Part model, mm, in its own coordinate system. A direction names the side the tool comes from. Round coordinates to 2 decimals unless told otherwise and drop trailing zeros. Loops run counter-clockwise (first coordinate to the right, second up) from the corner with the lowest first, then second, coordinate; pieces in that order, holes last. Notation, with made-up numbers: M -22.75,-1.75 L 9.25,-1.75 A18 cw 9.25,13.25 Z; hole C -14.5,68.25 d3. An arc over 180 degrees is marked long. Write each question's results on one line, items separated by ' | '.
from build123d import *

# Parameters (mm, degrees)
PROFILEBOSS_EXTRUDE1_DEPTH           = 270
SKETCH2_R                            = 2.3
LEDSTRIPMOUNTHOLESCUT_EXTRUDE1_DEPTH = 4.5
SKETCH3_R                            = 2.3
MOUNTINGHOLESCUT_EXTRUDE3_DEPTH      = 4.5
SKETCH4_W                            = 28
SKETCH4_H                            = 11.5
POWERCONNECTORCUT_EXTRUDE4_DEPTH     = 6.5


with BuildPart() as part:
    # Sketch1 → ProfileBoss-Extrude1 (new body)
    with BuildSketch(Plane(origin=(0, 0, 0), x_dir=(0, 0, -1), z_dir=(1, 0, 0))):
        with BuildLine():
            Line((0, 0), (2.499461553, 0))
            ThreePointArc((2.499461553, 0), (3.914055855, 0.585944145), (4.5, 2.000538447))
            Line((4.5, 2.000538447), (4.5, 3.5))
            Line((4.5, 3.5), (14.922539551, 8.36011001))
            Line((14.922539551, 8.36011001), (16.190394336, 5.641186649))
            ThreePointArc((16.190394336, 5.641186649), (17.700753359, 6.16912635), (18.340729536, 7.635528477))
            Line((18.340729536, 7.635528477), (18.340729536, 13.36011001))
            ThreePointArc((18.340729536, 13.36011001), (17.754943098, 14.774323572), (16.340729536, 15.36011001))
            Line((16.340729536, 15.36011001), (0, 15.36011001))
            Line((0, 15.36011001), (0, 0))
        make_face()
    extrude(amount=PROFILEBOSS_EXTRUDE1_DEPTH)

    # Sketch2 → LedStripMountHolesCut-Extrude1 (cut)
    with BuildSketch(Plane(origin=(0, 1.15127832, 0.536849897), x_dir=(1, 0, 0), z_dir=(0, -0.906307787036651, -0.4226182617406973))):
        with Locations(Location((36.15, -9.494933384, 0), (0, 0, 270))):
            Circle(SKETCH2_R)
        with Locations(Location((233.85, -11.307548958, 0), (0, 0, 270))):
            Circle(SKETCH2_R)
    extrude(amount=-LEDSTRIPMOUNTHOLESCUT_EXTRUDE1_DEPTH, mode=Mode.SUBTRACT)

    # Sketch3 → MountingHolesCut-Extrude3 (cut)
    with BuildSketch(Plane.XY):
        with Locations((50, 10.86011001)):
            Circle(SKETCH3_R)
        with Locations((220, 10.86011001)):
            Circle(SKETCH3_R)
    extrude(amount=-MOUNTINGHOLESCUT_EXTRUDE3_DEPTH, mode=Mode.SUBTRACT)

    # Sketch4 → PowerConnectorCut-Extrude4 (cut)
    with BuildSketch(Plane(origin=(0, 1.15127832, 0.536849897), x_dir=(1, 0, 0), z_dir=(0, -0.906307787036651, -0.4226182617406973))):
        with Locations((256, -11.307548958)):
            Rectangle(SKETCH4_W, SKETCH4_H)
        with Locations((14, -11.307548958)):
            Rectangle(SKETCH4_W, SKETCH4_H)
    extrude(amount=-POWERCONNECTORCUT_EXTRUDE4_DEPTH, mode=Mode.SUBTRACT)


solid = part.part
Item 1: Which spindle directions (+Z, -Z, +X, -X, +Y, -Y) get a long thin tool onto all of the face, cutting with end or side? Do faces 4 (the flat face through (220, 11, -4.5)), 5 (the flat face through (133.502, 5.896, -9.638)), 6 (the flat face through (270, 13, -7)), 7 (the flat face through (242, 9, -8)), 8 (the flat face through (13.804, 6.404, -3.146)). Say none if no direction does.
Filled sheet:
face 4: +Z | face 5: +X, -X, -Y | face 6: +Z, -Z, +X, +Y, -Y | face 7: +X | face 8: -X
Item 2: Two-plate mould, pull along Y, no slides. Class faces 1 (the flat face through (133, 15.36, -8)), 2 (the flat face through (233.882, 9.995, -7.78)), 3 (the flat face through (133, 10, -18.341)): +Y half, -Y half, draft (parallel to the pull), parting line (faces both ways), or undercut.
Filled sheet:
face 1: +Y half | face 2: undercut | face 3: draft
Item 3: Wall check: L1, parallel to X at y = 10.5, z = -3; L2, parallel to Y at x = 220, z = -0.9; L3, parallel to X at y = 12.75, z = -10. Give the ranges that are in metal, low to high.
Filled sheet:
L1: 0 to 47.73, 52.27 to 217.73, 222.27 to 270 | L2: 0 to 8.56, 13.16 to 15.36 | L3: 28 to 242
Item 4: Band-saw the part on A-A on x = 220. Give the cut face in (y, z).
Filled sheet:
outline: M 0,-2.5 A2 ccw 2,-4.5 L 3.5,-4.5 L 8.36,-14.92 L 5.64,-16.19 A2 ccw 7.64,-18.34 L 13.36,-18.34 A2 ccw 15.36,-16.34 L 15.36,0 L 13.16,0 L 13.16,-4.5 L 8.56,-4.5 L 8.56,0 L 0,0 Z
Item 5: Drop flat-ended pins along their axis: P1, Ø3.5, axis at x = 50, y = 10.5, coming from the +Z side; P2, Ø1, axis at x = 221.5, z = -3.5, coming from the -Y side; P3, Ø3, axis at y = 5, z = -10.5, coming from the +X side. Give the stop position or say it passes through.
Filled sheet:
P1: z = -4.5 | P2: y = 0.06 | P3: x = 242
Item 6: Band-saw the part on B-B on x = 44.5. Give the cut face in (y, z), and give its area (3 significant figures).
Filled sheet:
outline: M 0,-2.5 A2 ccw 2,-4.5 L 3.5,-4.5 L 8.36,-14.92 L 5.64,-16.19 A2 ccw 7.64,-18.34 L 13.36,-18.34 A2 ccw 15.36,-16.34 L 15.36,0 L 0,0 Z | area: 196 mm^2
